from build123d import *

# Parameters (mm, degrees)
SKETCH1_R           = 10
SKETCH1_W           = 46
SKETCH1_H           = 19.048435613
BOSS_EXTRUDE1_DEPTH = 46
CHAMFER1_SIZE       = 10
SKETCH2_R           = 9
BOSS_EXTRUDE2_DEPTH = 46
BOSS_EXTRUDE4_DEPTH = 10
SKETCH6_R           = 9.525638377
BOSS_EXTRUDE5_DEPTH = 10
SKETCH8_R           = 8.459669001
BOSS_EXTRUDE6_DEPTH = 50
DRAFT1_ANGLE        = 1
SKETCH9_R           = 14
SKETCH9_R_2         = 11
BOSS_EXTRUDE8_DEPTH = 40
DRAFT10_ANGLE       = 1.5
SKETCH12_W          = 62.404350154
SKETCH12_H          = 55.405731445
BOSS_EXTRUDE9_DEPTH = 10
FILLET1_R           = 10
FILLET2_R           = 10
SKETCH13_R          = 4
CUT_EXTRUDE3_DEPTH  = 10
DRAFT11_ANGLE       = 2
DRAFT12_ANGLE       = 4
DRAFT13_ANGLE       = 1
DRAFT14_ANGLE       = 1.5


# Read off the part's stored shape, not the designer's step: Draft7, Draft16
with BuildPart() as part:
    # Sketch1 → Boss-Extrude1 (new body)
    # profile 1 of 2: a face of its own
    with BuildSketch(Plane.XY):
        with BuildLine():
            Line((-23, 23), (-23, 0))
            ThreePointArc((-23, 0), (0, -23), (23, 0))
            Line((23, 0), (23, 23))
            Line((23, 23), (-23, 23))
        make_face()
        Circle(SKETCH1_R, mode=Mode.SUBTRACT)
    # profile 2 of 2: a face of its own
    with BuildSketch(Plane.XY):
        with Locations((0, 32.524217807)):
            Rectangle(SKETCH1_W, SKETCH1_H)
    extrude(amount=BOSS_EXTRUDE1_DEPTH)

    # Chamfer1
    chamfer1_edges = [part.edges().sort_by_distance(p)[0] for p in [
        (-23, 42.048435613, 23),
        (23, 42.048435613, 23),
        (0, 42.048435613, 46),
        (0, 42.048435613, 0),
    ]]
    chamfer(chamfer1_edges, length=CHAMFER1_SIZE)

    # Sketch2 → Boss-Extrude2 (add)
    with BuildSketch(Plane(origin=(0, 21.024217806, 0), x_dir=(1, 0, 0), z_dir=(0, 1, 0))):
        with Locations(Location((0, -22.756992406, 0), (0, 0, 270))):
            Circle(SKETCH2_R)
    extrude(amount=BOSS_EXTRUDE2_DEPTH)

    # Sketch5 → Boss-Extrude4 (add)
    with BuildSketch(Plane(origin=(0, 67.024217806, 0), x_dir=(1, 0, 0), z_dir=(0, 1, 0))):
        Polygon((10.943751373, -29.282952175), (11.123522631, -16.542405589), (0.179771258, -10.01644582), (-10.943751373, -16.231032637), (-11.123522631, -28.971579223), (-0.179771258, -35.497538992), align=None)
    extrude(amount=BOSS_EXTRUDE4_DEPTH)

    # Sketch6 → Boss-Extrude5 (add)
    with BuildSketch(Plane(origin=(0, 77.024217806, 0), x_dir=(1, 0, 0), z_dir=(0, 1, 0))):
        with Locations(Location((0, -22.484455751, 0), (0, 0, 270))):
            Circle(SKETCH6_R)
    extrude(amount=BOSS_EXTRUDE5_DEPTH)

    # Sketch8 → Boss-Extrude6 (add)
    with BuildSketch(Plane(origin=(0, 87.024217806, 0), x_dir=(1, 0, 0), z_dir=(0, 1, 0))):
        with Locations(Location((0, -22.484455751, 0), (0, 0, 270))):
            Circle(SKETCH8_R)
    extrude(amount=BOSS_EXTRUDE6_DEPTH)

    # Draft1
    draft1_faces = [part.faces().sort_by_distance(p)[0] for p in [
        (0, 112.024217806, 14.02478675),
    ]]
    draft(draft1_faces, Plane(origin=(0, 137.024217806, 22.484455751), x_dir=(0, 0, 1), z_dir=(0, 1, 0)), DRAFT1_ANGLE)

    # Draft7 outline → Draft7 (revolve)
    with BuildSketch(Plane.XY.offset(22.484455751)):
        Polygon((9.525638377, 87.024217806), (9.525638377, 96.316489669), (8.459669001, 137.024217806), (9.332422247, 87.024217806), align=None)
    revolve(axis=Axis((0, 0, 22.484455751), (0, 1, 0)))



with BuildPart() as body_2:
    # Sketch9 → Boss-Extrude8 (new body)
    with BuildSketch(Plane(origin=(0, 137.024217806, 0), x_dir=(1, 0, 0), z_dir=(0, 1, 0))):
        with Locations(Location((0, -22.484455751, 0), (0, 0, 270))):
            Circle(SKETCH9_R)
        with Locations(Location((0, -22.484455751, 0), (0, 0, 270))):
            Circle(SKETCH9_R_2, mode=Mode.SUBTRACT)
    extrude(amount=-BOSS_EXTRUDE8_DEPTH)

    # Draft10
    draft10_faces = [body_2.faces().sort_by_distance(p)[0] for p in [
        (0, 117.024217806, 8.484455751),
    ]]
    draft(draft10_faces, Plane(origin=(0, 137.024217806, 22.484455751), x_dir=(0, 0, 1), z_dir=(0, 1, 0)), DRAFT10_ANGLE)


with BuildPart() as part_1:
    add(part.part)

    add(body_2.part)  # Boss-Extrude9 merges body 2
    # Sketch12 → Boss-Extrude9 (add)
    with BuildSketch(Plane(origin=(0, 97.024217806, 0), x_dir=(-1, 0, 0), z_dir=(0, -1, 0))):
        with Locations((-0.437413669, -22.756992406)):
            Rectangle(SKETCH12_W, SKETCH12_H)
    extrude(amount=BOSS_EXTRUDE9_DEPTH)

    # Fillet1
    fillet1_edges = [part_1.edges().sort_by_distance(p)[0] for p in [
        (-30.764761408, 92.024217806, 50.459858128),
        (31.639588746, 92.024217806, -4.945873317),
        (31.639588746, 92.024217806, 50.459858128),
    ]]
    fillet(fillet1_edges, radius=FILLET1_R)

    # Fillet2
    fillet2_edges = [part_1.edges().sort_by_distance(p)[0] for p in [
        (-30.764761408, 92.024217806, -4.945873317),
    ]]
    fillet(fillet2_edges, radius=FILLET2_R)

    # Sketch13 → Cut-Extrude3 (cut)
    with BuildSketch(Plane(origin=(0, 97.024217806, 0), x_dir=(1, 0, 0), z_dir=(0, 1, 0))):
        with Locations(Location((-20.652282418, -42.41614068, 0), (0, 0, 270))):
            Circle(SKETCH13_R)
        with Locations(Location((21.744824706, -42.41614068, 0), (0, 0, 270))):
            Circle(SKETCH13_R)
        with Locations(Location((-20.652282418, -3.159218326, 0), (0, 0, 270))):
            Circle(SKETCH13_R)
        with Locations(Location((21.639588746, -3.159218326, 0), (0, 0, 270))):
            Circle(SKETCH13_R)
    extrude(amount=-CUT_EXTRUDE3_DEPTH, mode=Mode.SUBTRACT)

    # Draft11
    draft11_faces = [part_1.faces().sort_by_distance(p)[0] for p in [
        (0, 117.024217806, 7.960737319),
    ]]
    draft(draft11_faces, Plane(origin=(0, 137.024217806, 22.484455751), x_dir=(0, 0, 1), z_dir=(0, 1, 0)), DRAFT11_ANGLE)

    # Draft12
    draft12_faces = [part_1.faces().sort_by_distance(p)[0] for p in [
        (0, 117.024217806, 7.786040361),
    ]]
    draft(draft12_faces, Plane(origin=(0, 137.024217806, 22.484455751), x_dir=(0, 0, 1), z_dir=(0, 1, 0)), DRAFT12_ANGLE)

    # Draft13
    draft13_faces = [part_1.faces().sort_by_distance(p)[0] for p in [
        (0, 117.024217806, 7.085919512),
    ]]
    draft(draft13_faces, Plane(origin=(0, 137.024217806, 22.484455751), x_dir=(0, 0, 1), z_dir=(0, 1, 0)), DRAFT13_ANGLE)

    # Draft14
    draft14_faces = [part_1.faces().sort_by_distance(p)[0] for p in [
        (0, 117.024217806, 8.135354452),
    ]]
    draft(draft14_faces, Plane(origin=(0, 137.024217806, 22.484455751), x_dir=(0, 0, 1), z_dir=(0, 1, 0)), DRAFT14_ANGLE)

    # Draft16 outline → Draft16 (revolve, cut)
    with BuildSketch(Plane.XY.offset(22.484455751)):
        Polygon((14, 137.024217806), (12.250364385, 137.024217806), (15.047436863, 97.024217806), align=None)
    revolve(axis=Axis((0, 0, 22.484455751), (0, 1, 0)), mode=Mode.SUBTRACT)


solid = part_1.part
The model under review builds one solid part; all positions refer to its coordinate system, in mm. A direction names the side the tool comes from. Give positions to 0.01 mm unless a question says otherwise; leave off trailing zeros. Loops run counter-clockwise (first coordinate to the right, second up) from the corner with the lowest first, then second, coordinate; pieces in that order, holes last. Notation, with made-up numbers: (52.5, 50.25) -> (62.5, 50.25) arc R20 cw to (62.5, 85.25) -> close; hole circle Ø11 at (30.5, 25). An arc over 180 degrees is marked (long way). Answer as a JSON object with one key per item and string values. Group by question number.
Q1. Take a section at C-C (y = 15). Write out the cut boundary in (x, z), plus the area to 3 significant figures.
Q2. Take a section at A-A (y = -4.5). Write out the cut boundary in (x, z), plus the area to 3 significant figures.
Q3. Take a section at B-B (y = 125). Write out the cut boundary in (x, z), plus the area to 3 significant figures.
Q4. Draft analysis for pull direction Z (two halves, no side actions). For faces 1 (the flat face through (0, 137.024, 22)), 2 (the flat face through (1, 92, 50.46)), 3 (the cylindrical face through (25.6, 92.1, 2.6)), state which applies: pulls with the +Z half, pulls with the -Z half, needs draft (parallel to the pull), parting line crosses it, or undercut.
Q5. Wall thickness on line 1 along Y through (x, z) = (-3, -2); line 2 along Y through (x, z) = (16.5, 29); line 3 along Y through (x, z) = (1.5, 25.5): over which ranges is each line inside the solid? List them lowest first.
Q6. Tool access review of faces 4 (the flat face through (23, 16, 23)), 5 (the conical face through (8.562, 117.304, 19.788)), 6 (the flat face through (-0.32, 37.12, 40.93)), 7 (the flat face through (5.304, 71.954, 32.434)), 8 (the flat face through (17.93, 37.12, 22.68)): name each direction out of +Z, -Z, +X, -X, +Y, -Y from which nothing blocks a thin tool from reaching the whole face with its end or side.
Q7. Insertion check: pin 1 (10.5 mm diameter, centred on x = -20.65, z = 3.16, fed in from +Y); pin 2 (1.5 mm diameter, centred on y = 107, z = 6.5, fed in from +X); pin 3 (16.5 mm diameter, centred on x = -13.5, z = 9, fed in from -Y); pin 4 (4 mm diameter, centred on x = 16, y = 41, fed in from +Z). Each pin has a flat end and moves straight along its axis. Give the tip position at first contact, or say it passes through.
Answer below:
{
 "1": {"outline": "(-23, 0) -> (23, 0) -> (23, 46) -> (-23, 46) -> close", "area": "2,120 mm2"},
 "2": {"outline": "(-22.56, 0) -> (-8.93, 0) -> (-8.93, 46) -> (-22.56, 46) -> close; (8.93, 0) -> (22.56, 0) -> (22.56, 46) -> (8.93, 46) -> close", "area": "1,250 mm2"},
 "3": {"outline": "circle Ø26.18 at (0, 22.48); circle Ø17.55 at (0, 22.48); hole circle Ø22 at (0, 22.48)", "area": "400 mm2"},
 "4": {"face 1": "needs draft", "face 2": "pulls with the +Z half", "face 3": "undercut"},
 "5": {"line 1": "y = 87.02 to 97.02", "line 2": "y = -16.02 to 38.55, 87.02 to 97.02", "line 3": "y = -22.95 to -9.89, 9.89 to 137.02"},
 "6": {"face 4": "+Z, -Z, +X, -Y", "face 5": "+Y", "face 6": "+Z, +X, -X", "face 7": "+Z, +X", "face 8": "+Z, -Z, +X"},
 "7": {"pin 1": "stops at y = 97.02", "pin 2": "passes through", "pin 3": "stops at y = -22.39", "pin 4": "stops at z = 39.05"}
}
